```python
from build123d import *

# Parameters (mm, degrees)
F1_DEPTH  = 2
F2_W      = 96
F2_H      = 78
F3_DEPTH  = 4
F5_DEPTH  = 2
F6_R      = 1.25
F7_DEPTH  = 6
F8_R      = 2.25
F9_DEPTH  = 1.6
F11_R     = 1
F12_DEPTH = 1.5
F14_R     = 3
F15_DEPTH = 4
F16_R     = 1
F17_R     = 1.25
F18_DEPTH = 1
F19_R     = 0.75
F20_DEPTH = 4
F13_W     = 2.2
F13_H     = 4.2
F13_W_2   = 4.2
F21_W     = 4.2
F21_H     = 4.2
F22_DEPTH = 2


with BuildPart() as f1:
    # F0 (on Top) → F1 (new body)
    with BuildSketch(Plane.XY):
        with BuildLine():
            ThreePointArc((0, 2), (0.585786, 0.585786), (2, 0))
            Line((2, 0), (98, 0))
            ThreePointArc((98, 0), (99.414214, 0.585786), (100, 2))
            Line((100, 2), (100, 80))
            ThreePointArc((100, 80), (99.414214, 81.414214), (98, 82))
            Line((98, 82), (2, 82))
            ThreePointArc((2, 82), (0.585786, 81.414214), (0, 80))
            Line((0, 80), (0, 2))
        make_face()
    extrude(amount=F1_DEPTH)

    # F2 (on face) → F3 (join)
    with BuildSketch(Plane.XY.offset(2)):
        with BuildLine():
            ThreePointArc((2, 82), (0.585786, 81.414214), (0, 80))
            Line((0, 80), (0, 2))
            ThreePointArc((0, 2), (0.585786, 0.585786), (2, 0))
            Line((2, 0), (98, 0))
            ThreePointArc((98, 0), (99.414214, 0.585786), (100, 2))
            Line((100, 2), (100, 80))
            ThreePointArc((100, 80), (99.414214, 81.414214), (98, 82))
            Line((98, 82), (2, 82))
        make_face()
        with Locations((50, 41)):
            Rectangle(F2_W, F2_H, mode=Mode.SUBTRACT)
    extrude(amount=F3_DEPTH)

    # F4 (on face) → F5 (join)
    with BuildSketch(Plane.XY.offset(2)):
        with BuildLine():
            Line((2, 9), (2, 2))
            Line((2, 2), (9, 2))
            Line((9, 2), (9, 7))
            ThreePointArc((9, 7), (8.414214, 8.414214), (7, 9))
            Line((7, 9), (2, 9))
        make_face()
        with BuildLine():
            Line((9, 80), (2, 80))
            Line((2, 80), (2, 73))
            Line((2, 73), (7, 73))
            ThreePointArc((7, 73), (8.414214, 73.585786), (9, 75))
            Line((9, 75), (9, 80))
        make_face()
        with BuildLine():
            Line((91, 2), (98, 2))
            Line((98, 2), (98, 9))
            Line((98, 9), (93, 9))
            ThreePointArc((93, 9), (91.585786, 8.414214), (91, 7))
            Line((91, 7), (91, 2))
        make_face()
        with BuildLine():
            Line((98, 73), (98, 80))
            Line((98, 80), (91, 80))
            Line((91, 80), (91, 75))
            ThreePointArc((91, 75), (91.585786, 73.585786), (93, 73))
            Line((93, 73), (98, 73))
        make_face()
    extrude(amount=F5_DEPTH)

    # F6 (on face) → F7 (cut)
    with BuildSketch(Plane(origin=(0, 0, 0), x_dir=(1, 0, 0), z_dir=(0, 0, -1))):
        with Locations((94.5, -5.5)):
            Circle(F6_R)
        with Locations((94.5, -76.5)):
            Circle(F6_R)
        with Locations((5.5, -76.5)):
            Circle(F6_R)
        with Locations((5.5, -5.5)):
            Circle(F6_R)
    extrude(amount=-F7_DEPTH, mode=Mode.SUBTRACT)

    # F8 (on face) → F9 (cut)
    with BuildSketch(Plane(origin=(0, 0, 0), x_dir=(1, 0, 0), z_dir=(0, 0, -1))):
        with Locations((5.5, -76.5)):
            Circle(F8_R)
        with Locations((5.5, -5.5)):
            Circle(F8_R)
        with Locations((94.5, -5.5)):
            Circle(F8_R)
        with Locations((94.5, -76.5)):
            Circle(F8_R)
    extrude(amount=-F9_DEPTH, mode=Mode.SUBTRACT)

    # F11
    f11_edges = [f1.edges().sort_by_distance(p)[0] for p in [
        (50, 82, 0),
    ]]
    fillet(f11_edges, radius=F11_R)

    # F10 (on face) → F12 (join)
    with BuildSketch(Plane.XY.offset(2)):
        with BuildLine():
            ThreePointArc((73, 27), (73.292893, 26.292893), (74, 26))
            Line((74, 26), (77, 26))
            ThreePointArc((77, 26), (77.707107, 26.292893), (78, 27))
            Line((78, 27), (78, 55))
            ThreePointArc((78, 55), (77.707107, 55.707107), (77, 56))
            Line((77, 56), (74, 56))
            ThreePointArc((74, 56), (73.292893, 55.707107), (73, 55))
            Line((73, 55), (73, 27))
        make_face()
    extrude(amount=F12_DEPTH)

    # F14 (on face) → F15 (join)
    with BuildSketch(Plane.XY.offset(2)):
        with Locations((46.65, 75.25)):
            Circle(F14_R)
        with Locations((46.65, 6.75)):
            Circle(F14_R)
    extrude(amount=F15_DEPTH)

    # F16
    f16_edges = [f1.edges().sort_by_distance(p)[0] for p in [
        (43.65, 75.25, 6),
        (43.65, 6.75, 6),
    ]]
    fillet(f16_edges, radius=F16_R)

    # F17 (on face) → F18 (cut)
    with BuildSketch(Plane(origin=(0, 0, 0), x_dir=(1, 0, 0), z_dir=(0, 0, -1))):
        with Locations((46.65, -75.25)):
            Circle(F17_R)
        with Locations((46.65, -6.75)):
            Circle(F17_R)
    extrude(amount=-F18_DEPTH, mode=Mode.SUBTRACT)

    # F19 (on face) → F20 (cut)
    with BuildSketch(Plane(origin=(0, 0, 1), x_dir=(1, 0, 0), z_dir=(0, 0, -1))):
        with Locations((46.65, -6.75)):
            Circle(F19_R)
        with Locations((46.65, -75.25)):
            Circle(F19_R)
    extrude(amount=-F20_DEPTH, mode=Mode.SUBTRACT)

    # F13 (on face) + F21 (on face) → F22 (cut)
    with BuildSketch(Plane.XY.offset(2)):
        with Locations((65, 75.9)):
            Rectangle(F13_W, F13_H)
        with Locations((65, 6.1)):
            Rectangle(F13_W, F13_H)
        with Locations((34, 6.1)):
            Rectangle(F13_W_2, F13_H)
    with BuildSketch(Plane.XY.offset(2)):
        with Locations((34, 75.9)):
            Rectangle(F21_W, F21_H)
    extrude(amount=-F22_DEPTH, mode=Mode.SUBTRACT)


solid = f1.part
```
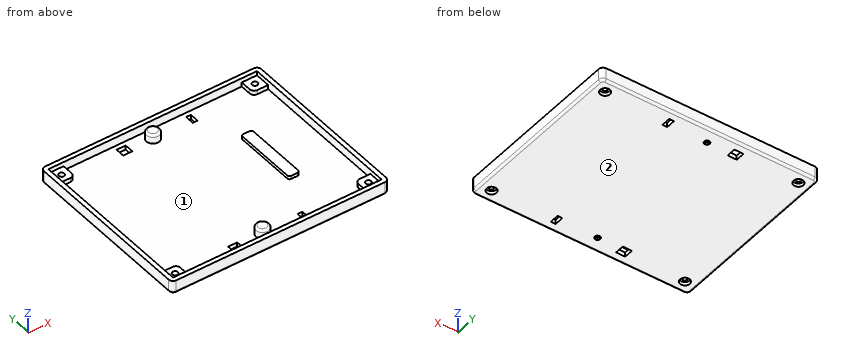
Check sheet for the modelled part. Datum: model origin and axes. Units: mm. Face numbers are marked on the shaded views. Give positions to 0.01 mm unless a question says otherwise; leave off trailing zeros. Write each loop counter-clockwise with the first axis right and the second up, starting at its lowest first coordinate (ties: lowest second). Pieces come first, ordered by that corner, then holes.
Item 1: Cross-section at B-B (y = 21). Enter the section's corners in (x, z).
Item 2: Cross-section at C-C (y = 42.5). Enter the section's corners in (x, z), and give its area (3 significant figures).
Item 3: Scan lines: L1, parallel to Y at x = 94.5, z = 1; L2, parallel to X at y = 5.5, z = 1; L3, parallel to Y at x = 46.65, z = 2.9. Record each from-to range of solid material in increasing order.
Item 4: Cross-section at A-A (x = 5.5). Count the separate pieces of the cut face and the enclosed holes in it, and give its area (3 significant figures).
Item 5: Draft check along Y on the marked faces 1 and 2. Enter one of: released by +Y, released by -Y, zero draft, split by the parting line, or undercut.
Item 6: Gauge pin test, flat ends, axial feed: pin 1 (1.3 mm diameter, centred on x = 94.5, y = 75.5, fed in from -Z); pin 2 (2 mm diameter, centred on x = 96, y = 75.5, fed in from +Z); pin 3 (12 mm diameter, centred on x = 72.5, y = 40, fed in from +Z); pin 4 (2 mm diameter, centred on x = 47, y = 7.5, fed in from -Z). Record the tip position at first contact, or that the pin passes through.
Report:
1. outline: (0, 1) arc R1 ccw to (1, 0) - (99, 0) arc R1 ccw to (100, 1) - (100, 6) - (98, 6) - (98, 2) - (2, 2) - (2, 6) - (0, 6) - close
2. outline: (0, 1) arc R1 ccw to (1, 0) - (99, 0) arc R1 ccw to (100, 1) - (100, 6) - (98, 6) - (98, 2) - (78, 2) - (78, 3.5) - (73, 3.5) - (73, 2) - (2, 2) - (2, 6) - (0, 6) - close
2. area: 223 mm2
3. L1: y = 0 to 3.25, 7.75 to 74.25, 78.75 to 82
3. L2: x = 0 to 3.25, 7.75 to 31.9, 36.1 to 63.9, 66.1 to 92.25, 96.75 to 100
3. L3: y = 0 to 2, 3.75 to 6, 7.5 to 9.75, 72.25 to 74.5, 76 to 78.25, 80 to 82
4. separate pieces: 3
4. enclosed holes: 0
4. area: 181 mm2
5. face 1: undercut
5. face 2: zero draft
6. pin 1: stops at z = 1.6
6. pin 2: stops at z = 4
6. pin 3: stops at z = 3.5
6. pin 4: stops at z = 0
